Check sheet for the modelled part. Datum: model origin and axes. Units: mm. A direction names the side the tool comes from. Coordinates: 2 decimals unless noted, no trailing zeros. Order: outer loops, then holes, each group sorted by start corner. A loop starts at its lowest first (then second) coordinate and runs counter-clockwise, first axis right, second up.
1. Set-up check for faces 4 (the cylindrical face through (-9.974, 2.364, 7.148)), 5 (the cylindrical face through (4.1, 27.1, -6.4)): record each of +Z, -Z, +X, -X, +Y, -Y from which the full face is reachable in a straight line by a thin tool's end or side.
2. Cross-section at D-D (z = 0). Enter the section's corners in (x, y).
3. Cross-section at B-B (x = 8.5). Enter the section's corners in (y, z).
4. Gauge pin test, flat ends, axial feed: pin 1 Ø1.5 at (y, z) = (17.5, 6.5) entering from -X; pin 2 Ø6 at (y, z) = (13.5, -10) entering from +X; pin 3 Ø1 at (x, z) = (-5.5, -9) entering from +Y; pin 4 Ø7 at (x, z) = (0, 0) entering from +Y. Record the tip position at first contact, or that the pin passes through.
5. Thickness scan on line 1 (Z direction, x = -8.5, y = 3); line 2 (Z direction, x = -0.25, y = 10.5); line 3 (Y direction, x = -1.25, z = 9.75). Record the ranges inside material, lowest first.
6. Cross-section at C-C (x = 0). Enter the section's corners in (y, z), then the cut area to 3 significant figures.
7. Draft check along X on faces 1 (the flat face through (-3, -0.2, -3)), 2 (the cylindrical face through (3.815, 24.45, -1.201)), 3 (the flat face through (-12.5, 2, 0)). Enter one of: released by +X, released by -X, zero draft, split by the parting line, or undercut.
8. Cross-section at A-A (z = -8.5). Enter the section's corners in (x, y).
```python
from build123d import *

# Parameters (mm, degrees)
CYLINDER006_R          = 2
CYLINDER006_DEPTH      = 10
CYLINDER007_R          = 2
CYLINDER007_DEPTH      = 10
CYLINDER005_R          = 2
CYLINDER005_DEPTH      = 10
CYLINDER004_R          = 2
CYLINDER004_DEPTH      = 10
CYLINDER003_R          = 4
CYLINDER003_DEPTH      = 60
CYLINDER002_R          = 7.6
CYLINDER002_DEPTH      = 45
BOX_W                  = 25
BOX_H                  = 25
BOX_DEPTH              = 5.2
CUT004_PLACEMENT_ANGLE = 90


with BuildPart() as cylinder006:
    # Cylinder006 → Cylinder006 (new body)
    with BuildSketch(Plane(origin=(21, 21, -2), x_dir=(1, 0, 0), z_dir=(0, 0, 1))):
        Circle(CYLINDER006_R)
    extrude(amount=CYLINDER006_DEPTH)


with BuildPart() as cylinder007:
    # Cylinder007 → Cylinder007 (new body)
    with BuildSketch(Plane(origin=(21, 4, -2), x_dir=(1, 0, 0), z_dir=(0, 0, 1))):
        Circle(CYLINDER007_R)
    extrude(amount=CYLINDER007_DEPTH)


with BuildPart() as cylinder005:
    # Cylinder005 → Cylinder005 (new body)
    with BuildSketch(Plane(origin=(4, 21, -2), x_dir=(1, 0, 0), z_dir=(0, 0, 1))):
        Circle(CYLINDER005_R)
    extrude(amount=CYLINDER005_DEPTH)


with BuildPart() as cylinder004:
    # Cylinder004 → Cylinder004 (new body)
    with BuildSketch(Plane(origin=(4, 4, -2), x_dir=(1, 0, 0), z_dir=(0, 0, 1))):
        Circle(CYLINDER004_R)
    extrude(amount=CYLINDER004_DEPTH)


with BuildPart() as cylinder003:
    # Cylinder003 → Cylinder003 (new body)
    with BuildSketch(Plane(origin=(12.5, 12.5, -7), x_dir=(1, 0, 0), z_dir=(0, 0, 1))):
        Circle(CYLINDER003_R)
    extrude(amount=CYLINDER003_DEPTH)


with BuildPart() as cylinder002:
    # Cylinder002 → Cylinder002 (new body)
    with BuildSketch(Plane(origin=(12.5, 12.5, 5), x_dir=(1, 0, 0), z_dir=(0, 0, 1))):
        Circle(CYLINDER002_R)
    extrude(amount=CYLINDER002_DEPTH)


with BuildPart() as cut004:
    # Box → Box (new body)
    with BuildSketch(Plane.XY):
        with Locations((12.5, 12.5)):
            Rectangle(BOX_W, BOX_H)
    extrude(amount=BOX_DEPTH)

    # Fusion: union Cylinder002
    add(cylinder002.part)

    # Cut: cut Cylinder003
    add(cylinder003.part, mode=Mode.SUBTRACT)

    # Cut001: cut Cylinder004
    add(cylinder004.part, mode=Mode.SUBTRACT)

    # Cut002: cut Cylinder005
    add(cylinder005.part, mode=Mode.SUBTRACT)

    # Cut003: cut Cylinder007
    add(cylinder007.part, mode=Mode.SUBTRACT)

    # Cut004: cut Cylinder006
    add(cylinder006.part, mode=Mode.SUBTRACT)


with BuildPart() as cut004_1:
    # Cut004 placement: moved
    add(cut004.part.moved(Location((-12.5, -0.2, 12.5))).rotate(Axis((-12.5, -0.2, 12.5), (-1, 0, 0)), CUT004_PLACEMENT_ANGLE))


solid = cut004_1.part
```
Data:
1. face 4: +Y, -Y
1. face 5: +Y
2. outline: (-12.5, -0.2) - (-4, -0.2) - (-4, 49.8) - (-7.6, 49.8) - (-7.6, 5) - (-12.5, 5) - close; (4, -0.2) - (12.5, -0.2) - (12.5, 5) - (7.6, 5) - (7.6, 49.8) - (4, 49.8) - close
3. outline: (-0.2, -12.5) - (5, -12.5) - (5, -10.5) - (-0.2, -10.5) - close; (-0.2, -6.5) - (5, -6.5) - (5, 6.5) - (-0.2, 6.5) - close; (-0.2, 10.5) - (5, 10.5) - (5, 12.5) - (-0.2, 12.5) - close
4. pin 1: stops at x = -4.97
4. pin 2: stops at x = 2.96
4. pin 3: stops at y = 5
4. pin 4: passes through
5. line 1: z = -12.5 to -10.5, -6.5 to 6.5, 10.5 to 12.5
5. line 2: z = -7.6 to -3.99, 3.99 to 7.6
5. line 3: y = -0.2 to 5
6. outline: (-0.2, -12.5) - (5, -12.5) - (5, -7.6) - (49.8, -7.6) - (49.8, -4) - (-0.2, -4) - close; (-0.2, 4) - (49.8, 4) - (49.8, 7.6) - (5, 7.6) - (5, 12.5) - (-0.2, 12.5) - close
6. area: 411 mm2
7. face 1: zero draft
7. face 2: undercut
7. face 3: released by -X
8. outline: (-12.5, -0.2) - (-10.5, -0.2) - (-10.5, 5) - (-12.5, 5) - close; (-6.5, -0.2) - (6.5, -0.2) - (6.5, 5) - (-6.5, 5) - close; (10.5, -0.2) - (12.5, -0.2) - (12.5, 5) - (10.5, 5) - close
